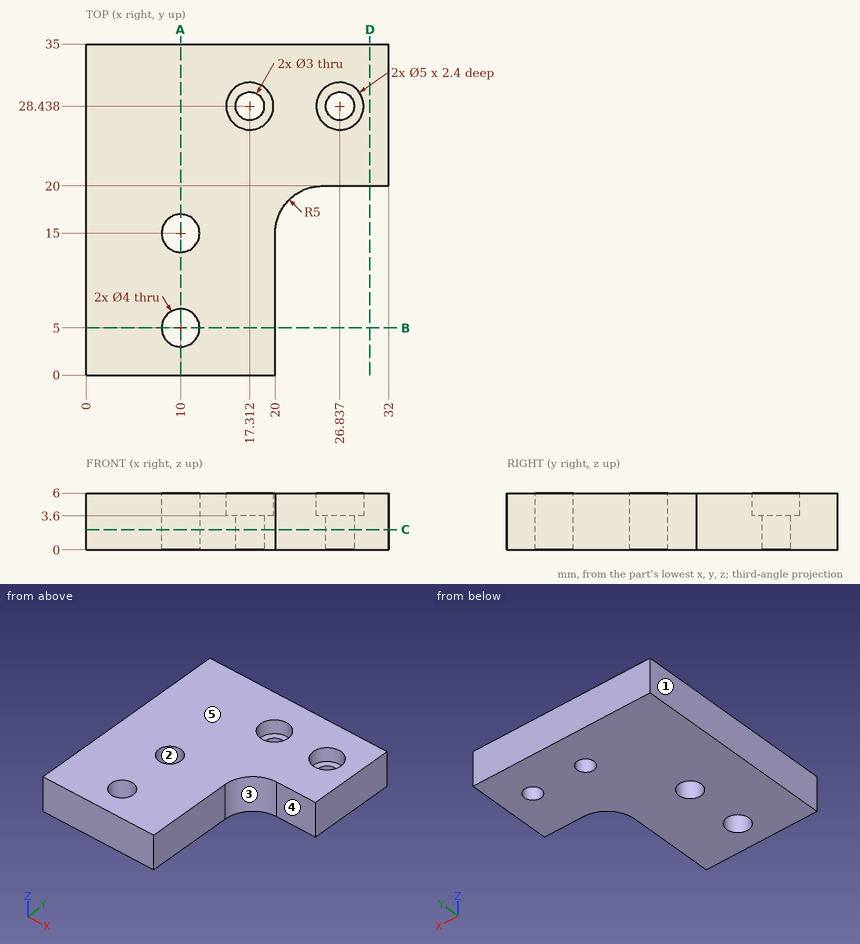
Geometry check sheet. Reference: drawing and pictorial views, mm from the part's lowest x, y, z. A direction names the side the tool comes from. Give positions to 0.01 mm unless a question says otherwise; leave off trailing zeros. Loops run counter-clockwise (first coordinate to the right, second up) from the corner with the lowest first, then second, coordinate; pieces in that order, holes last. Notation, with made-up numbers: (71.25, 40) - (87.25, 40) arc R13 cw to (87.25, 57) - close; hole circle Ø7 at (47.25, 30). An arc over 180 degrees is marked (long way). One line per question, with ' | ' between items. Start each with the question number.
1. Set-up check for the marked faces 4 and 5: record each of +Z, -Z, +X, -X, +Y, -Y from which the full face is reachable in a straight line by a thin tool's end or side.
2. Cross-section at A-A, the plane x = 10. Enter the section's corners in (y, z).
3. Gauge pin test, flat ends, axial feed: pin 1 Ø3 at (x, z) = (27, 1.5) entering from -Y; pin 2 Ø1.5 at (x, y) = (28, 29) entering from +Z. Record the tip position at first contact, or that the pin passes through.
4. Cross-section at C-C, the plane z = 2.15. Enter the section's corners in (x, y).
5. Material ranges on line 1 along Y through (x, z) = (27, 1.85); line 2 along X through (y, z) = (27.5, 0.45) (1 decimal); line 3 along Y through (x, z) = (10.5, 0.65) (1 decimal), recorded low to high. Write a range as [from, to].
6. Draft check along Y on the marked faces 1, 2 and 3. Enter one of: released by +Y, released by -Y, zero draft, split by the parting line, or undercut.
7. Cross-section at D-D, the plane x = 30. Enter the section's corners in (y, z), plus the area to 3 significant figures.
8. Cross-section at B-B, the plane y = 5. Enter the section's corners in (x, z).
Check result:
1) face 4: +Z, -Z, +X, -Y | face 5: +Z, +X, -X, +Y, -Y
2) outline: (0, 0) - (3, 0) - (3, 6) - (0, 6) - close; (7, 0) - (13, 0) - (13, 6) - (7, 6) - close; (17, 0) - (35, 0) - (35, 6) - (17, 6) - close
3) pin 1: stops at y = 20 | pin 2: stops at z = 3.6
4) outline: (0, 0) - (20, 0) - (20, 15) arc R5 cw to (25, 20) - (32, 20) - (32, 35) - (0, 35) - close; hole circle Ø4 at (10, 5); hole circle Ø4 at (10, 15); hole circle Ø3 at (17.31, 28.44); hole circle Ø3 at (26.84, 28.44)
5) line 1: y = [20, 26.95], [29.93, 35] | line 2: x = [0, 16.1], [18.5, 25.7], [28, 32] | line 3: y = [0, 3.1], [6.9, 13.1], [16.9, 35]
6) face 1: zero draft | face 2: undercut | face 3: released by -Y
7) outline: (20, 0) - (35, 0) - (35, 6) - (20, 6) - close | area: 90.0 mm2
8) outline: (0, 0) - (8, 0) - (8, 6) - (0, 6) - close; (12, 0) - (20, 0) - (20, 6) - (12, 6) - close
